Autodesk Inventor part; units mm, degrees
ref_plane "YZ Plane" through (0, 0, 0) normal (1, 0, 0) x (0, 1, 0)
ref_plane "XZ Plane" through (0, 0, 0) normal (0, 1, 0) x (-1, 0, 0)
ref_plane "XY Plane" through (0, 0, 0) normal (0, 0, 1) x (1, 0, 0)
sketch "Sketch2" plane through (0, 0, 0) normal (0, 1, 0) x (-1, 0, 0)
  line L0 (0, 0) -> (10, 0)
  line L1 (10, 0) -> (10, -13)
  line L2 (10, -13) -> (0, -13)
  line L3 (0, -13) -> (0, 0)
  line L4 (10, -4.3333) -> (3, -4.3333)
  line L5 (3, -4.3333) -> (3, -8.6667)
  line L6 (3, -8.6667) -> (10, -8.6667)
  line L7 (10, -8.6667) -> (10, -4.3333)
  dimension "d4" = 13
  dimension "d5" = 10
  dimension "d6" = 4.3333
  dimension "d7" = 7
  dimension "d8" = 4.3333
extrude "Extrusion2" add sketch "Sketch2" along normal blind 6 contours L0 L1 L4 L5 L6 L2 L3
sketch "Sketch3" plane through (-10, 0, 0) normal (0, 0, 1) x (1, 0, 0)
  line L0 (7, 9) -> (7, -3) construction
  line L1 (4, 9) -> (4, -3)
  line L2 (10, -3) -> (10, 9)
  arc A0 (10, 9) -> (4, 9) centre (7, 9) ccw
  arc A1 (4, -3) -> (10, -3) centre (7, -3) ccw
  circle A2 centre (7, 9) radius 1.5
  circle A3 centre (7, -3) radius 1.5
  line L3 (10, 0) -> (10, 6)
  line L4 (0, 6) -> (10, 6)
  line L5 (0, 0) -> (10, 0)
  point P0 (7, 3)
  dimension "d11" = 12
  dimension "d12" = 6
  dimension "d13" = 3
  dimension "d14" = 3
  dimension "d15" = 3
  dimension "d16" = 6
extrude "Extrusion3" add sketch "Sketch3" against normal blind 2
sketch "Sketch4" plane through (0, 0, -13) normal (1, 0, 0) x (0, 0, -1)
  circle A0 centre (-10.5, 4.5) radius 0.5
  line L0 (-8.6667, 0) -> (-8.6667, 6)
  line L1 (-8.6667, 5.6316) -> (-8.6667, 4.1699)
  circle A1 centre (-10.5, 3.5) radius 0.5
  circle A2 centre (-10.5, 2.5) radius 0.5
  circle A3 centre (-10.5, 1.5) radius 0.5
  line L2 (-11, 6) -> (0, 6)
  line L3 (-11, 0) -> (0, 0)
  line L4 (-11, 0) -> (-11, -3)
  point P0 (-13, 0)
  dimension "d19" = 1
  dimension "d22" = 1
  dimension "d27" = 1.5
  dimension "d28" = 3
  dimension "d29" = 6
  dimension "d30" = 0.5
extrude "Extrusion4" add sketch "Sketch4" along normal blind 2
sketch "Sketch5" plane through (-10, 0, -8.6667) normal (0, 0, 1) x (1, 0, 0)
  circle A0 centre (3.5, 3) radius 0.25
  circle A1 centre (4.5, 3) radius 0.25
  line L0 (7, 0) -> (7, 6)
  line L1 (0, 6) -> (7, 6)
  point P0 (10, 0)
  dimension "d33" = 0.5
  dimension "d34" = 0.5
  dimension "d35" = 1
  dimension "d36" = 2.5
  dimension "d37" = 3
extrude "Extrusion5" cut sketch "Sketch5" against normal blind 1
equation "\"d6\" = 0.333333 * d4"
equation "\"d8\" = 0.333333 * d4"
equation "\"d14\" = d13"
equation "\"d27\" = -0.5 * d28 + 0.5 * d29"
equation "\"d37\" = 0.5 * d16"
properties part number "InkrementalisOptikaiErzekelo" material "UHMW, Black"
Work out the finished part from the listing and answer in its coordinate system (mm). A direction names the side the tool comes from. Give positions to 0.01 mm unless a question says otherwise; leave off trailing zeros. Write each loop counter-clockwise with the first axis right and the second up, starting at its lowest first coordinate (ties: lowest second). Pieces come first, ordered by that corner, then holes.
Q1. Given pin 1 (2.5 mm diameter, centred on x = -3, y = 9, fed in from -Z); pin 2 (4 mm diameter, centred on x = -2.5, y = -4, fed in from -Z); pin 3 (4 mm diameter, centred on y = -1, z = -11.5, fed in from +X); pin 4 (2 mm diameter, centred on y = 7.5, z = -1, fed in from -X), each flat-ended and moving along its own axis, determine where each tip first touches the part or whether it passes through.
Answer:
pin 1: passes through
pin 2: stops at z = -2
pin 3: stops at x = 0
pin 4: stops at x = -6
Q2. The part is cut by section C-C on y = 10.25. Give the vertices of the cut face in (x, z).
Answer:
outline: (-5.73, -2) - (-3.83, -2) - (-3.83, 0) - (-5.73, 0) - close; (-2.17, -2) - (-0.27, -2) - (-0.27, 0) - (-2.17, 0) - close
Q3. The part is cut by section A-A on x = -8.25. Give the vertices of the cut face in (y, z), and give its area (3 significant figures).
Answer:
outline: (0, -13) - (6, -13) - (6, -8.67) - (0, -8.67) - close; (0, -4.33) - (6, -4.33) - (6, 0) - (0, 0) - close
area: 52.0 mm2
Q4. The part is cut by section D-D on z = -4.75. Give the vertices of the cut face in (x, y).
Answer:
outline: (-3, 0) - (0, 0) - (0, 6) - (-3, 6) - close
Q5. For a pull along Y with two mould halves and no side action, classify faces 5 (the face through (-3, -6, -1)), 6 (the face through (-2.31, 7.67, -0.99)), 7 (the face through (-6, 2, -8.667)) as released by +Y, released by -Y, zero draft, split by the parting line, or undercut.
Answer:
face 5: released by -Y
face 6: undercut
face 7: zero draft
Q6. The part is cut by section B-B on y = 5.25. Give the vertices of the cut face in (x, z).
Answer:
outline: (-10, -13) - (0, -13) - (0, 0) - (-10, 0) - (-10, -4.33) - (-3, -4.33) - (-3, -8.67) - (-10, -8.67) - close
Q7. Straight lines are drawn through the part: L1, parallel to Z at x = -3.5, y = 2.5; L2, parallel to Y at x = -3, z = -1.55; L3, parallel to Y at x = -0.25, z = -12.25. For each, find the intervals that lie inside material, in ascending order.
Answer:
L1: z = -13 to -8.67, -4.33 to 0
L2: y = -6 to -4.5, -1.5 to 7.5, 10.5 to 12
L3: y = 0 to 6
Q8. A tool of negligible diameter and unlimited length cuts with its end or side. For faces 1 (the face through (-3, 3, -6)), 2 (the face through (-6, 8, -1)), 3 (the face through (-3, 7, -2)), 4 (the face through (-6, -1, -1)), from which of +Z, -Z, +X, -X, +Y, -Y can it reach the whole face along a straight path? Write none if from no direction.
Answer:
face 1: -X, +Y, -Y
face 2: +Z, -Z, -X, +Y
face 3: -Z, +X, -X, +Y
face 4: +Z, -Z, -X, -Y
